Work out the finished part from the listing and answer in its coordinate system (mm). Coordinates: 2 decimals unless noted, no trailing zeros. Loops run counter-clockwise (first coordinate to the right, second up) from the corner with the lowest first, then second, coordinate; pieces in that order, holes last. Notation, with made-up numbers: M 57.25,-35 L 62.25,-35 A22 cw 62.25,-8 Z; hole C -16.75,38.5 d2. An arc over 180 degrees is marked long. Write each question's results on one line, items separated by ' | '.
Autodesk Inventor part; units mm, degrees
ref_plane "YZ Plane" through (0, 0, 0) normal (1, 0, 0) x (0, 1, 0)
ref_plane "XZ Plane" through (0, 0, 0) normal (0, 1, 0) x (-1, 0, 0)
ref_plane "XY Plane" through (0, 0, 0) normal (0, 0, 1) x (1, 0, 0)
sketch "Sketch1" plane through (0, 0, 0) normal (0, 0, 1) x (1, 0, 0)
  line L0 (66.802, 0) -> (66.802, 38.1)
  line L1 (0, 38.1) -> (0, 0)
  line L2 (9.525, 31.75) -> (57.277, 31.75) construction
  line L3 (57.277, 31.75) -> (57.277, 6.35) construction
  line L4 (57.277, 6.35) -> (9.525, 6.35) construction
  line L5 (9.525, 6.35) -> (9.525, 31.75) construction
  circle A0 centre (9.525, 31.75) radius 3.3782
  circle A1 centre (9.525, 6.35) radius 3.3782
  circle A2 centre (57.277, 31.75) radius 3.3782
  circle A3 centre (57.277, 6.35) radius 3.3782
  line L6 (0, 0) -> (0, -25.4)
  line L7 (0, -25.4) -> (66.802, -25.4)
  line L8 (66.802, -25.4) -> (66.802, 0)
  line L9 (0, 38.1) -> (0, 76.2)
  line L10 (0, 76.2) -> (66.802, 76.2)
  line L11 (66.802, 76.2) -> (66.802, 38.1)
  point P0 (0, 0)
  dimension "d0" = 38.1
  dimension "d1" = 66.802
  dimension "d2" = 25.4
  dimension "d3" = 47.752
  dimension "d4" = 9.525
  dimension "d6" = 6.7564
  dimension "d7" = 6.7564
  dimension "d8" = 6.7564
  dimension "d9" = 6.7564
  dimension "d14" = 6.35
  dimension "d15" = 9.525
  dimension "d17" = 25.4
  dimension "d18" = 101.6
extrude "Extrusion1" add sketch "Sketch1" along normal blind 3.175
sketch "Sketch4" plane through (0, 0, 3.175) normal (0, 0, 1) x (1, 0, 0)
  line L0 (66.802, -25.4) -> (66.802, 76.2)
  line L1 (0, -25.4) -> (66.802, -25.4)
  circle A0 centre (41.402, -12.7) radius 2.0701
  circle A1 centre (41.402, 63.5) radius 2.0701
  point P0 (0, 0)
  dimension "d31" = 4.1402
  dimension "d32" = 25.4
  dimension "d33" = 12.7
  dimension "d34" = 4.1402
  dimension "d35" = 76.2
  dimension "d36" = 25.4
extrude "Extrusion4" cut sketch "Sketch4" against normal blind 25.4
fillet "Fillet1" radius 6.35 4 edges at (0, 76.2, 1.5875) (66.802, 76.2, 1.5875) (0, -25.4, 1.5875) (66.802, -25.4, 1.5875)
sketch "Sketch5" plane through (0, 0, 3.175) normal (0, 0, 1) x (1, 0, 0)
  line L0 (0, 69.85) -> (0, -19.05)
  arc A0 (0, -19.05) -> (6.35, -25.4) centre (6.35, -19.05) ccw
  line L1 (6.35, -25.4) -> (60.452, -25.4)
  line L2 (0, 0) -> (19.05, 0)
  line L3 (19.05, 0) -> (19.05, -25.4)
  point P0 (0, 0)
  dimension "d40" = 25.4
  dimension "d41" = 19.05
extrude "Extrusion5" cut sketch "Sketch5" against normal blind 25.4
equation "\"d4\" = -0.5 * d3 + 0.5 * d1"
properties part number "Aluminum Plate (0.125)" material "Aluminum 6061"
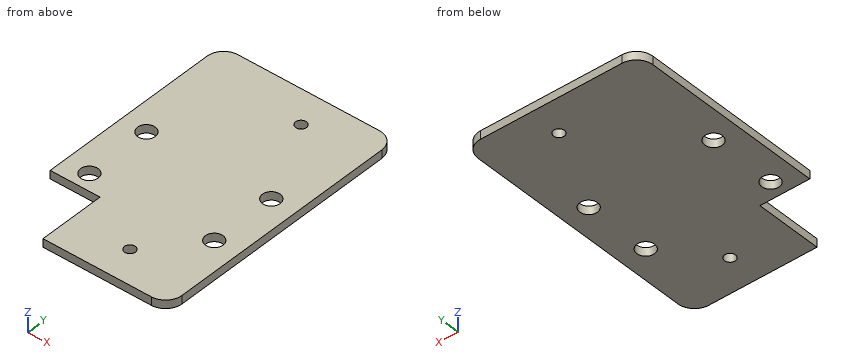
1) Given pin 1 Ø1.6 at (x, z) = (6, 1) entering from -Y, flat-ended and moving along its own axis, determine where the tip first touches the part or whether it passes through.
Check result:
pin 1: y = 0
2) Find section B-B, the plane y = 6.35. Give the vertices of the cut face in (x, z) (3 decimals), and give its area (3 significant figures).
Check result:
outline: M 0,0 L 6.147,0 L 6.147,3.175 L 0,3.175 Z; M 12.903,0 L 53.899,0 L 53.899,3.175 L 12.903,3.175 Z; M 60.655,0 L 66.802,0 L 66.802,3.175 L 60.655,3.175 Z | area: 169 mm^2
3) Find section C-C, the plane z = 1.3. Give the vertices of the cut face in (x, y) (3 decimals).
Check result:
outline: M 0,0 L 19.05,0 L 19.05,-25.4 L 60.452,-25.4 A6.35 ccw 66.802,-19.05 L 66.802,69.85 A6.35 ccw 60.452,76.2 L 6.35,76.2 A6.35 ccw 0,69.85 Z; hole C 9.525,6.35 d6.756; hole C 9.525,31.75 d6.756; hole C 41.402,-12.7 d4.14; hole C 41.402,63.5 d4.14; hole C 57.277,6.35 d6.756; hole C 57.277,31.75 d6.756
4) Find section A-A, the plane y = 63.5. Give the vertices of the cut face in (x, z) (3 decimals), and give its area (3 significant figures).
Check result:
outline: M 0,0 L 39.332,0 L 39.332,3.175 L 0,3.175 Z; M 43.472,0 L 66.802,0 L 66.802,3.175 L 43.472,3.175 Z | area: 199 mm^2
5) Straight lines are drawn through the part: probe 1 along X at (y, z) = (4, 1); probe 2 along Y at (x, z) = (40.5, 2.2); probe 3 along Y at (x, z) = (41, 1.3). For each, find the intervals that lie inside material, in ascending order. Write a range as [from, to].
Check result:
probe 1: [0, 7.1], [11.95, 54.85], [59.7, 66.8] | probe 2: [-25.4, -14.56], [-10.84, 61.64], [65.36, 76.2] | probe 3: [-25.4, -14.73], [-10.67, 61.47], [65.53, 76.2]
6) Find section D-D, the plane y = 33.5. Give the vertices of the cut face in (x, z) (3 decimals), and give its area (3 significant figures).
Check result:
outline: M 0,0 L 6.635,0 L 6.635,3.175 L 0,3.175 Z; M 12.415,0 L 54.387,0 L 54.387,3.175 L 12.415,3.175 Z; M 60.167,0 L 66.802,0 L 66.802,3.175 L 60.167,3.175 Z | area: 175 mm^2
